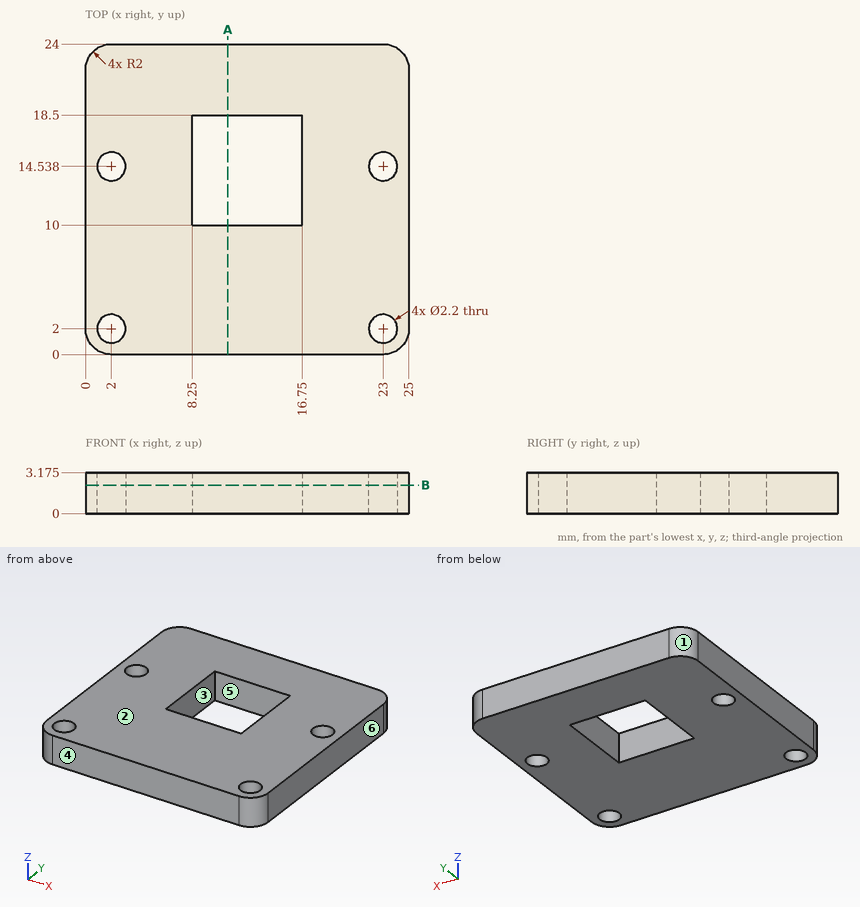
Design review of the part shown in the three views and the two pictorial views. Dimensions are in mm from the part's minimum x, y and z. A direction names the side the tool comes from. Give positions to 0.01 mm unless a question says otherwise; leave off trailing zeros. Loops run counter-clockwise (first coordinate to the right, second up) from the corner with the lowest first, then second, coordinate; pieces in that order, holes last. Notation, with made-up numbers: (7, 19) -> (40, 19) arc R19 cw to (40, 30) -> close; hole circle Ø5 at (68.25, 58). An arc over 180 degrees is marked (long way). One line per item, written item: value.
Q1. We need section A-A on x = 11. Give the boundary of the cut face in (y, z) (3 decimals).
Numbers:
outline: (0, 0) -> (10, 0) -> (10, 3.175) -> (0, 3.175) -> close; (18.5, 0) -> (24, 0) -> (24, 3.175) -> (18.5, 3.175) -> close
Q2. For pin 1 Ø1.8 at (x, y) = (23, 2) entering from -Z (3 decimals), flat-tipped, find the tip position at first contact; note if it passes through.
Numbers:
pin 1: passes through
Q3. For L1, parallel to Y at x = 23, z = 1.65; L2, parallel to Y at x = 13.5, z = 1.15; L3, parallel to X at y = 12.5, z = 1, list the stretches that pass through material, from the lowest coordinate up.
Numbers:
L1: y = 0 to 0.9, 3.1 to 13.44, 15.64 to 24
L2: y = 0 to 10, 18.5 to 24
L3: x = 0 to 8.25, 16.75 to 25
Q4. We need section B-B on z = 2.2. Give the boundary of the cut face in (x, y).
Numbers:
outline: (0, 2) arc R2 ccw to (2, 0) -> (23, 0) arc R2 ccw to (25, 2) -> (25, 22) arc R2 ccw to (23, 24) -> (2, 24) arc R2 ccw to (0, 22) -> close; hole circle Ø2.2 at (2, 2); hole circle Ø2.2 at (2, 14.54); hole (8.25, 10) -> (16.75, 10) -> (16.75, 18.5) -> (8.25, 18.5) -> close; hole circle Ø2.2 at (23, 2); hole circle Ø2.2 at (23, 14.54)
Q5. Draft analysis for pull direction Y (two halves, no side actions). For the marked faces 1, 2, 3 and 4, state which applies: pulls with the +Y half, pulls with the -Y half, needs draft (parallel to the pull), parting line crosses it, or undercut.
Numbers:
face 1: pulls with the +Y half
face 2: needs draft
face 3: undercut
face 4: pulls with the -Y half
Q6. Machinability: for the marked faces 5 and 6, which of the approach directions +Z, -Z, +X, -X, +Y, -Y give a long, thin tool a straight path to every point of the face, cutting with its end or side? Answer none if there is none.
Numbers:
face 5: +Z, -Z
face 6: +Z, -Z, +X, +Y, -Y
